Geometry check sheet. Reference: drawing and pictorial views, mm from the part's lowest x, y, z. A direction names the side the tool comes from. Give positions to 0.01 mm unless a question says otherwise; leave off trailing zeros. Loops run counter-clockwise (first coordinate to the right, second up) from the corner with the lowest first, then second, coordinate; pieces in that order, holes last. Notation, with made-up numbers: (42, -39.75) -> (66, -39.75) arc R15 cw to (66, -33.75) -> close; hole circle Ø11 at (38.5, 5.25). An arc over 180 degrees is marked (long way). One line per item, written item: value. Start each with the question number.
(1) Gauge pin test, flat ends, axial feed: pin 1 Ø4.5 at (y, z) = (20, 7.5) entering from +X; pin 2 Ø3.5 at (x, z) = (10.5, 7) entering from +Y. Record the tip position at first contact, or that the pin passes through.
(2) Sectioned sample at C-C, the plane y = 10.5. Record the cut outline in (x, z), then the cut area to 3 significant figures.
(3) Scan lines: line 1 along X through (y, z) = (8, 7.5); line 2 along Y through (x, z) = (4.45, 7.5); line 3 along Y through (x, z) = (16.5, 12.75). Record each from-to range of solid material in increasing order. Write a range as from..to.
(4) Draft check along Z on the marked faces 3, 4 and 5. Enter one of: pulls with the +Z half, pulls with the -Z half, needs draft (parallel to the pull), parting line crosses it, or undercut.
(5) Sectioned sample at D-D, the plane x = 2.25. Record the cut outline in (y, z), then the cut area to 3 significant figures.
(6) Sectioned sample at B-B, the plane x = 12. Record the cut outline in (y, z), then the cut area to 3 significant figures.
(7) Sectioned sample at A-A, the plane z = 7.5. Record the cut outline in (x, y).
(8) Tool access check on the marked faces 1 and 2. Record the directions out of +Z, -Z, +X, -X, +Y, -Y that give a thin tool (end or side, any length) a straight path to the whole face; none if there is none.
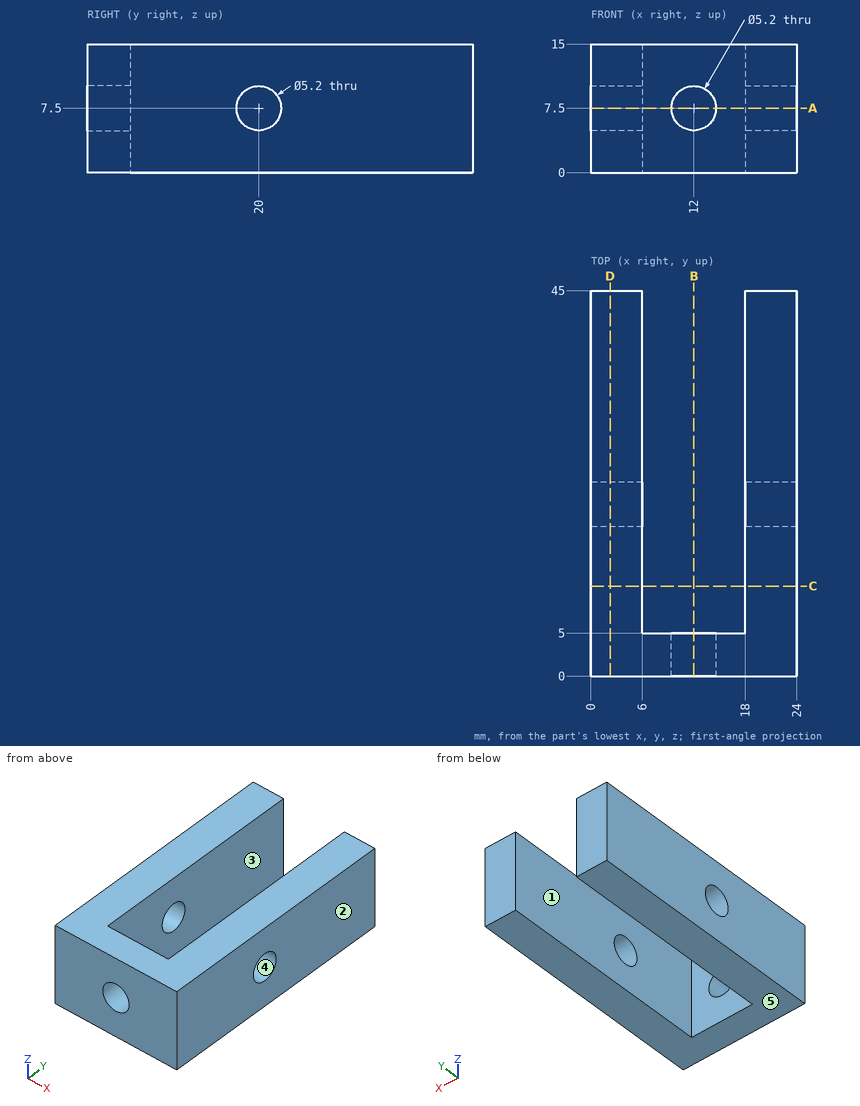
Calculated:
1. pin 1: passes through
1. pin 2: stops at y = 5
2. outline: (0, 0) -> (6, 0) -> (6, 15) -> (0, 15) -> close; (18, 0) -> (24, 0) -> (24, 15) -> (18, 15) -> close
2. area: 180 mm2
3. line 1: x = 0..6, 18..24
3. line 2: y = 0..17.4, 22.6..45
3. line 3: y = 0..5
4. face 3: needs draft
4. face 4: undercut
4. face 5: pulls with the -Z half
5. outline: (0, 0) -> (45, 0) -> (45, 15) -> (0, 15) -> close; hole circle Ø5.2 at (20, 7.5)
5. area: 654 mm2
6. outline: (0, 0) -> (5, 0) -> (5, 4.9) -> (0, 4.9) -> close; (0, 10.1) -> (5, 10.1) -> (5, 15) -> (0, 15) -> close
6. area: 49.0 mm2
7. outline: (0, 0) -> (9.4, 0) -> (9.4, 5) -> (6, 5) -> (6, 17.4) -> (0, 17.4) -> close; (0, 22.6) -> (6, 22.6) -> (6, 45) -> (0, 45) -> close; (14.6, 0) -> (24, 0) -> (24, 17.4) -> (18, 17.4) -> (18, 5) -> (14.6, 5) -> close; (18, 22.6) -> (24, 22.6) -> (24, 45) -> (18, 45) -> close
8. face 1: +Z, -Z, +Y
8. face 2: +Z, -Z, +X, +Y, -Y
